Source: CAD feature listing. Evaluate the final solid. Frame: model axes, mm. Round coordinates to 2 decimals unless told otherwise and drop trailing zeros. Order: outer loops, then holes, each group sorted by start corner. A loop starts at its lowest first (then second) coordinate and runs counter-clockwise, first axis right, second up. Notation, with made-up numbers: M 61,21 L 75,21 A12 cw 75,28 Z; hole C -24.75,39 d7. An arc over 180 degrees is marked long. Answer as CSV lines item,"result". Start each with the question number.
Item 1: Section query D-D on z = 172. Return the cut outline in (x, y), plus the area to 3 significant figures.
Item 2: Section query A-A on z = 81.5. Return the cut outline in (x, y), plus the area to 3 significant figures.
Item 3: First-contact query: P1, Ø6, axis at x = -75, y = 33.5, coming from the +Z side; P2, Ø4.5, axis at x = 89.5, y = 231, coming from the +Z side; P3, Ø8, axis at y = 189.5, z = 98.5, coming from the -X side. Flat tips, straight axial feed; report the tip coordinate or a pass-through.
Item 4: Line query: line 1 (Z direction, x = -28, y = 39); line 2 (X direction, y = 68, z = -96.5); line 3 (Z direction, x = -157, y = 100). Output: solid intervals per line, ascending. Write a range as [from, to].
Item 5: Section query B-B on y = 45.5. Return the cut outline in (x, z).
Item 6: Section query C-C on y = 90. Return the cut outline in (x, z).
from build123d import *

# Parameters (mm, degrees)
REVOLVE_1_ANGLE     = 180
SHELL_1_T           = -1
SKETCH_2_W          = 20
SKETCH_2_H          = 220
CUT_EXTRUDE_1_DEPTH = 434.012701892


with BuildPart() as part:
    # Эскиз1 → Повернуть1 (revolve)
    with BuildSketch(Plane(origin=(0, 0, 0), x_dir=(1, 0, 0), z_dir=(0, 1, 0))):
        with BuildLine():
            Line((-250, 0), (250, 0))
            ThreePointArc((250, 0), (0, 250), (-250, 0))
        make_face()
    revolve(axis=Axis((-250, 0, 0), (1, 0, 0)), revolution_arc=REVOLVE_1_ANGLE)

    # Оболочка1
    shell_1_openings = [part.faces().sort_by_distance(p)[0] for p in [
        (0, 0, 0),
    ]]
    offset(amount=SHELL_1_T, openings=shell_1_openings)

    # Эскиз2 → Вырез-Вытянуть1 (cut, through all)
    with BuildSketch(Plane(origin=(0, 0, 0), x_dir=(1, 0, 0), z_dir=(0, 1, 0))):
        with Locations((-90, -140)):
            Rectangle(SKETCH_2_W, SKETCH_2_H)
        with Locations((90, -140)):
            Rectangle(SKETCH_2_W, SKETCH_2_H)
    extrude(amount=CUT_EXTRUDE_1_DEPTH, mode=Mode.SUBTRACT)


solid = part.part
Results:
1,outline,"M -181.43,0 L -180.05,0 A180.05 cw -100,149.72 L -100,151.38 A181.43 ccw Z; M -80,161.3 A180.05 cw 80,161.3 L 80,162.84 A181.43 ccw -80,162.84 Z; M 100,149.72 A180.05 cw 180.05,0 L 181.43,0 A181.43 ccw 100,151.38 Z"
1,area,"720 mm^2"
2,outline,"M -236.34,0 L -235.28,0 A235.28 cw -100,212.98 L -100,214.14 A236.34 ccw Z; M -80,221.27 A235.28 cw 80,221.27 L 80,222.39 A236.34 ccw -80,222.39 Z; M 100,212.98 A235.28 cw 235.28,0 L 236.34,0 A236.34 ccw 100,214.14 Z"
2,area,"738 mm^2"
3,P1,"z = 237.14"
3,P2,"z = 30"
3,P3,"x = -136.31"
4,line 1,"[-245.35, -244.33], [244.33, 245.35]"
4,line 2,"[-220.37, -219.24], [219.24, 220.37]"
4,line 3,"[-166.89, -165.38], [165.38, 166.89]"
5,outline,"M -100,223.45 L -100,224.57 A245.82 ccw long 100,224.57 L 100,223.45 A244.81 cw long Z; M -80,231.37 A244.81 cw 80,231.37 L 80,232.44 A245.82 ccw -80,232.44 Z"
6,outline,"M -100,209.53 L -100,210.71 A233.24 ccw long 100,210.71 L 100,209.53 A232.17 cw long Z; M -80,217.95 A232.17 cw 80,217.95 L 80,219.09 A233.24 ccw -80,219.09 Z"
